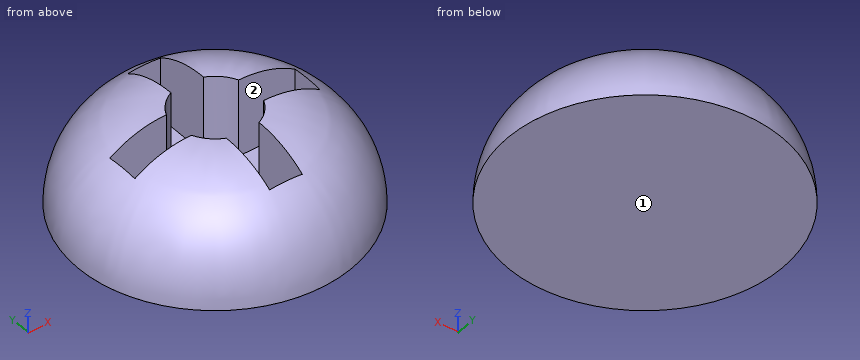
Autodesk Inventor part; units mm, degrees
ref_plane "YZ Plane" through (0, 0, 0) normal (1, 0, 0) x (0, 1, 0)
ref_plane "XZ Plane" through (0, 0, 0) normal (0, 1, 0) x (-1, 0, 0)
ref_plane "XY Plane" through (0, 0, 0) normal (0, 0, 1) x (1, 0, 0)
sketch "Sketch1" plane through (0, 0, 0) normal (0, 0, 1) x (1, 0, 0)
  circle A0 centre (-3.4351, -7.3738) radius 1.5
  circle A1 centre (-3.4351, -7.3738) radius 4.4749
  point P0 (0, 0)
extrude "Extrusion1" add sketch "Sketch1" along normal blind 3.175 contours A0 | A1
fillet "Fillet1" radius 3.175 1 edges at (-7.91, -7.3738, 3.175)
sketch "Sketch2" plane through (-3.4351, -7.3738, 3.175) normal (0, 0, 1) x (1, 0, 0)
  circle A0 centre (0, 0) radius 1.2999 construction
  line L0 (-6.0004, 0) -> (5.9052, 0) construction
  line L1 (0.0173, 5.7893) -> (0.0173, -4.6347) construction
  line L2 (1.1846, 0.5352) -> (3.0338, 0.5352)
  line L3 (3.0338, 0.5352) -> (3.0338, 0)
  line L4 (1.1846, -0.5352) -> (3.0338, -0.5352)
  line L5 (3.0338, -0.5352) -> (3.0338, 0)
  line L6 (-0.5352, 1.1846) -> (-0.5352, 3.0338)
  line L7 (-0.5352, 3.0338) -> (0, 3.0338)
  line L8 (0.5352, 1.1846) -> (0.5352, 3.0338)
  line L9 (0.5352, 3.0338) -> (0, 3.0338)
  line L10 (-1.1846, -0.5352) -> (-3.0338, -0.5352)
  line L11 (-3.0338, -0.5352) -> (-3.0338, 0)
  line L12 (-1.1846, 0.5352) -> (-3.0338, 0.5352)
  line L13 (-3.0338, 0.5352) -> (-3.0338, 0)
  line L14 (0.5352, -1.1846) -> (0.5352, -3.0338)
  line L15 (0.5352, -3.0338) -> (0, -3.0338)
  line L16 (-0.5352, -1.1846) -> (-0.5352, -3.0338)
  line L17 (-0.5352, -3.0338) -> (0, -3.0338)
  arc A1 (1.1846, 0.5352) -> (0.5352, 1.1846) centre (0, 0) ccw
  arc A2 (-0.5352, 1.1846) -> (-1.1846, 0.5352) centre (0, 0) ccw
  arc A3 (-1.1846, -0.5352) -> (-0.5352, -1.1846) centre (0, 0) ccw
  arc A4 (0.5352, -1.1846) -> (1.1846, -0.5352) centre (0, 0) ccw
  point P0 (3.4351, 7.3738)
  dimension "d5" = 360
extrude "Extrusion2" cut sketch "Sketch2" against normal blind 2.54
properties part number "Bolt1"
The model under review builds one solid part; all positions refer to its coordinate system, in mm. Face numbers are marked on the shaded views. Give positions to 0.01 mm unless a question says otherwise; leave off trailing zeros. Write item = value, one per line. Start each with the question number.
(1) For pin 1 Ø0.9 at (y, z) = (-7.5, 1.5) entering from +X; pin 2 Ø0.9 at (x, z) = (-1, 2.5) entering from -Y; pin 3 Ø0.9 at (y, z) = (-5.5, 1.5) entering from -X, all flat-tipped, find the tip position at first contact; note any pin that passes through.
(2) Draft analysis for pull direction X (two halves, no side actions). For the marked faces 1 and 2, state which applies: +X half, -X half, draft (parallel to the pull), parting line (faces both ways), or undercut.
(3) For L1, parallel to Z at x = -2, y = -7.5 (3 decimals); L2, parallel to Y at x = -1.25, z = 0.9; L3, parallel to Y at x = -4.5, z = 2.6, list the stretches that pass through material, from the lowest coordinate up. Write a range as from..to.
Returned:
q1.pin_1 = 0.86
q1.pin_2 = -10.31
q1.pin_3 = -7.39
q2.face_1 = draft
q2.face_2 = undercut
q3.L1 = 0..0.635
q3.L2 = -11.13..-7.91, -6.84..-3.62
q3.L3 = -10.31..-8.12, -6.63..-4.44
